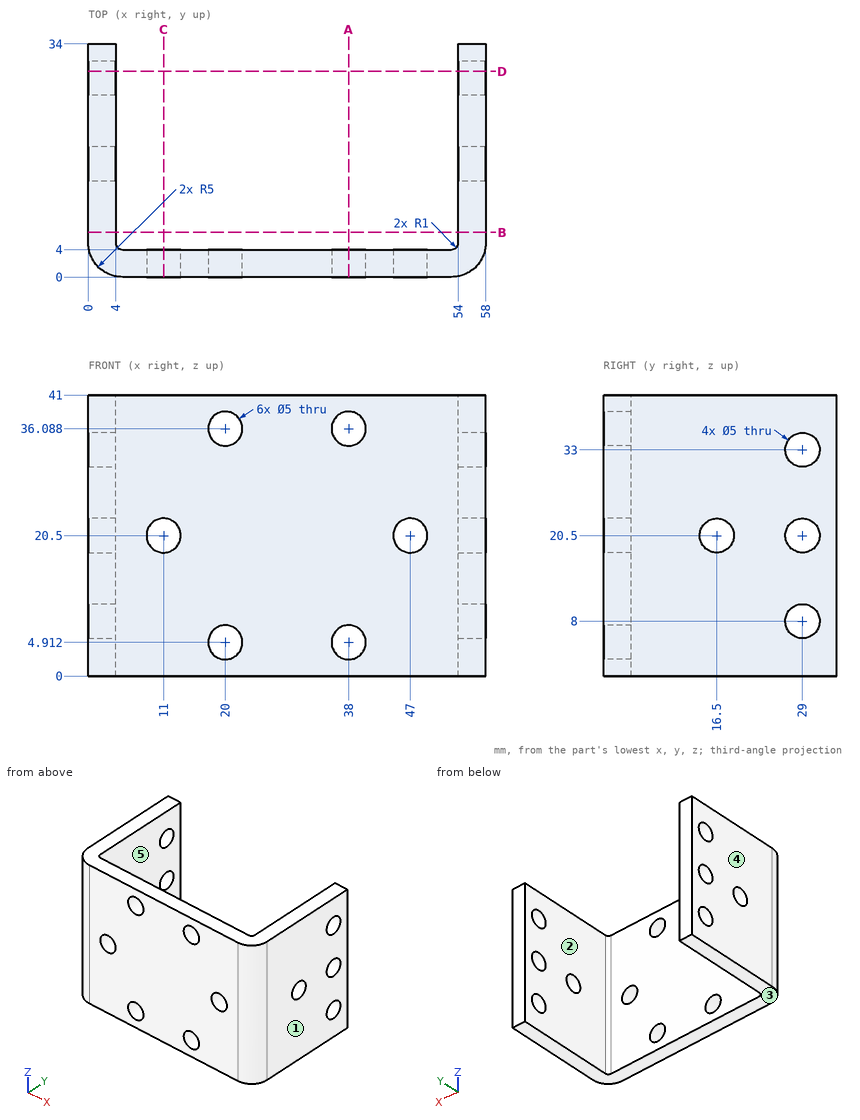
Could you check a few things on this drawing? It's one solid part, dimensions in mm from its lowest x, y, z. A direction names the side the tool comes from. Give positions to 0.01 mm unless a question says otherwise; leave off trailing zeros. Order: outer loops, then holes, each group sorted by start corner. A loop starts at its lowest first (then second) coordinate and runs counter-clockwise, first axis right, second up. Notation, with made-up numbers: (-2, -11.5) - (24, -11.5) arc R20 ccw to (24, 26.5) - close; hole circle Ø5 at (-7, 56). An arc over 180 degrees is marked (long way). One line per item, written item: value. Start each with the question number.
1. Imagine slicing it at C-C on x = 11. List the corners of the cut face in (y, z) for me.
2. Imagine slicing it at B-B on y = 6.5. List the corners of the cut face in (x, z) for me, plus the area to 3 significant figures.
3. Imagine slicing it at D-D on y = 30. Give the number of separate pieces and of enclosed holes in the cut face, plus the area to 3 significant figures.
4. If I drill on probe 1 along Z at (x, y) = (38, 1); probe 2 along X at (y, z) = (2, 37); probe 3 along X at (y, z) = (31.5, 29), over which ranges is the centre line in solid material (lowest first)?
5. For P1, Ø3, axis at x = 10.5, z = 17, coming from the +Y side; P2, Ø12, axis at x = 22.5, y = 13, coming from the +Z side, each with a flat end and sliding along its axis, tell me the tip position at first contact or that it passes through.
6. Thinking about a two-plate mould opening in X: for the marked faces 1, 2 and 3, which applies, +X half, -X half, draft (parallel to the pull), parting line (faces both ways), or undercut?
7. Imagine slicing it at A-A on x = 38. List the corners of the cut face in (y, z) for me.
8. For the marked faces 4 and 5, which set-ups out of +Z, -Z, +X, -X, +Y, -Y let a thin tool reach every point of the face, with its end or its side?
Values:
1. outline: (0, 0) - (4, 0) - (4, 18) - (0, 18) - close; (0, 23) - (4, 23) - (4, 41) - (0, 41) - close
2. outline: (0, 0) - (4, 0) - (4, 41) - (0, 41) - close; (54, 0) - (58, 0) - (58, 41) - (54, 41) - close
2. area: 328 mm²
3. separate pieces: 8
3. enclosed holes: 0
3. area: 218 mm²
4. probe 1: 0 to 2.41, 7.41 to 33.59, 38.59 to 41
4. probe 2: 1 to 17.67, 22.33 to 35.67, 40.33 to 57
4. probe 3: 0 to 4, 54 to 58
5. P1: y = 4
5. P2: through
6. face 1: +X half
6. face 2: undercut
6. face 3: draft
7. outline: (0, 0) - (4, 0) - (4, 2.41) - (0, 2.41) - close; (0, 7.41) - (4, 7.41) - (4, 33.59) - (0, 33.59) - close; (0, 38.59) - (4, 38.59) - (4, 41) - (0, 41) - close
8. face 4: +Z, -Z, -X, +Y, -Y
8. face 5: +Z, -Z, +Y
